Can you work these out from the model? Positions are in its coordinate system, mm. Give positions to 0.01 mm unless a question says otherwise; leave off trailing zeros. Loops run counter-clockwise (first coordinate to the right, second up) from the corner with the lowest first, then second, coordinate; pieces in that order, holes last. Notation, with made-up numbers: (-6.75, -34.75) -> (-0.75, -34.75) arc R31 cw to (-0.75, 4.25) -> close; hole circle Ø4 at (-3, -8). An arc over 180 degrees is marked (long way). Use CSV: the item, a comma, the result in double quotes.
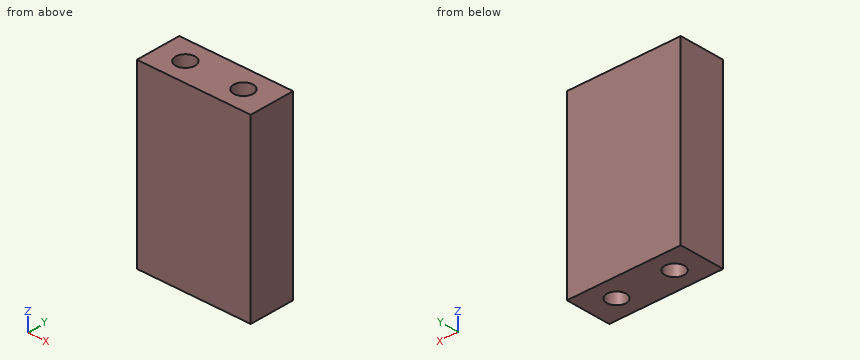
from build123d import *

# Parameters (mm, degrees)
ESQUISSE1_W                = 20
ESQUISSE1_H                = 8
BOSS_EXTRU_1_DEPTH         = 31.5
D_GAGEMENT_M31_D           = 3.4
R_P_TITION_LIN_AIRE1_COUNT = 2
R_P_TITION_LIN_AIRE1_PITCH = 10.2


with BuildPart() as part:
    # Esquisse1 → Boss.-Extru.1 (new body)
    with BuildSketch(Plane.XY):
        with Locations((-7.314758755, -1.171717172)):
            Rectangle(ESQUISSE1_W, ESQUISSE1_H)
    extrude(amount=BOSS_EXTRU_1_DEPTH)

    # Dégagement M31 (through all)
    with Locations(Plane.XY.offset(31.5)):
        with Locations((-2.314758755, -1.171717172)):
            d_gagement_m31 = Hole(D_GAGEMENT_M31_D / 2)

    # Répétition linéaire1: Dégagement M31 ×2
    with Locations(*[(-i * R_P_TITION_LIN_AIRE1_PITCH, 0, 0) for i in range(1, R_P_TITION_LIN_AIRE1_COUNT)]):
        add(d_gagement_m31, mode=Mode.SUBTRACT)


solid = part.part
(1) If I drill on L1, parallel to X at y = -1.25, z = 14.5; L2, parallel to X at y = -0.25, z = 29.5; L3, parallel to Y at x = -3, z = 14, over which ranges is the centre line in solid material (lowest first)? Write a range as from..to.
Answer sheet:
L1,"x = -17.31..-14.21, -10.82..-4.01, -0.62..2.69"
L2,"x = -17.31..-13.94, -11.09..-3.74, -0.89..2.69"
L3,"y = -5.17..-2.73, 0.38..2.83"
(2) If we section it at A-A, the plane x = -3.25: Write out the boundary of the cut face in (y, z), then the cut area to 3 significant figures.
Answer sheet:
outline,"(-5.17, 0) -> (-2.59, 0) -> (-2.59, 31.5) -> (-5.17, 31.5) -> close; (0.25, 0) -> (2.83, 0) -> (2.83, 31.5) -> (0.25, 31.5) -> close"
area,"163 mm2"
(3) If we section it at C-C, the plane z = 18: Write out the boundary of the cut face in (x, y).
Answer sheet:
outline,"(-17.31, -5.17) -> (2.69, -5.17) -> (2.69, 2.83) -> (-17.31, 2.83) -> close; hole circle Ø3.4 at (-12.51, -1.17); hole circle Ø3.4 at (-2.31, -1.17)"
(4) If we section it at B-B, the plane y = -0.5: Write out the boundary of the cut face in (x, z).
Answer sheet:
outline,"(-17.31, 0) -> (-14.08, 0) -> (-14.08, 31.5) -> (-17.31, 31.5) -> close; (-10.95, 0) -> (-3.88, 0) -> (-3.88, 31.5) -> (-10.95, 31.5) -> close; (-0.75, 0) -> (2.69, 0) -> (2.69, 31.5) -> (-0.75, 31.5) -> close"
